Verification items for this drawing (mm, ordinates from the low corner). Coordinates: 2 decimals unless noted, no trailing zeros. Loops run counter-clockwise (first coordinate to the right, second up) from the corner with the lowest first, then second, coordinate; pieces in that order, holes last.
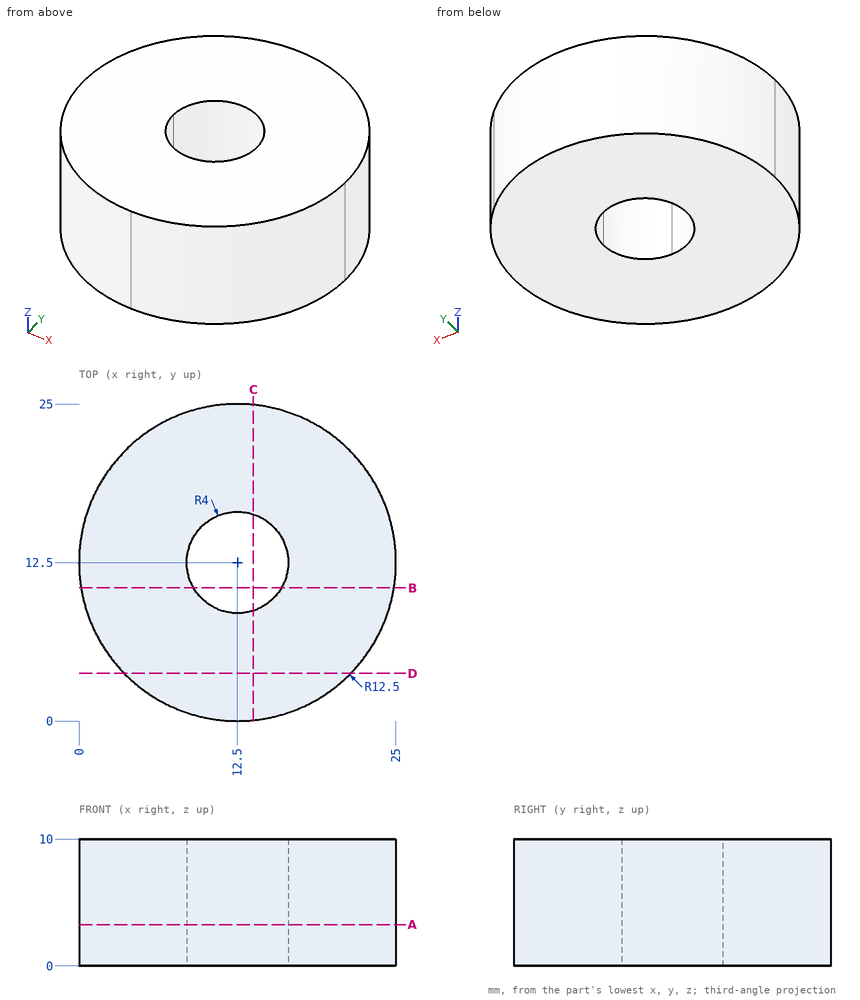
(1) Gauge pin test, flat ends, axial feed: P1, Ø1.5, axis at y = 21.5, z = 5.5, coming from the +X side; P2, Ø1, axis at y = 13.5, z = 6, coming from the +X side; P3, Ø1.5, axis at x = 3, z = 5.5, coming from the +Y side. Record the tip position at first contact, or that the pin passes through.
(2) Section check A-A, the plane z = 3.25. Enter the section's corners in (x, y), plus the area to 3 significant figures.
(3) Section check D-D, the plane y = 3.75. Enter the section's corners in (x, z).
(4) Scan lines: line 1 along Y through (x, z) = (12.5, 7); line 2 along X through (y, z) = (15.5, 2.75); line 3 along Y through (x, z) = (16, 0.5). Record each from-to range of solid material in increasing order.
(5) Section check B-B, the plane y = 10.5. Enter the section's corners in (x, z), plus the area to 3 significant figures.
(6) Section check C-C, the plane x = 13.75. Enter the section's corners in (y, z).
Determined:
1. P1: stops at x = 21.89
1. P2: stops at x = 24.99
1. P3: stops at y = 21.43
2. outline: circle Ø25 at (12.5, 12.5); hole circle Ø8 at (12.5, 12.5)
2. area: 441 mm2
3. outline: (3.57, 0) - (21.43, 0) - (21.43, 10) - (3.57, 10) - close
4. line 1: y = 0 to 8.5, 16.5 to 25
4. line 2: x = 0.37 to 9.85, 15.15 to 24.63
4. line 3: y = 0.5 to 10.56, 14.44 to 24.5
5. outline: (0.16, 0) - (9.04, 0) - (9.04, 10) - (0.16, 10) - close; (15.96, 0) - (24.84, 0) - (24.84, 10) - (15.96, 10) - close
5. area: 177 mm2
6. outline: (0.06, 0) - (8.7, 0) - (8.7, 10) - (0.06, 10) - close; (16.3, 0) - (24.94, 0) - (24.94, 10) - (16.3, 10) - close
